Work out the finished part from the listing and answer in its coordinate system (mm). A direction names the side the tool comes from. Give positions to 0.01 mm unless a question says otherwise; leave off trailing zeros. Write each loop counter-clockwise with the first axis right and the second up, starting at its lowest first coordinate (ties: lowest second). Pieces come first, ordered by that corner, then holes. Notation, with made-up numbers: (34, 28) -> (87, 28) arc R25 cw to (87, 65) -> close; hole circle Ø8 at (34.5, -22.75). An arc over 180 degrees is marked (long way). Use a Markdown table: item, result. Add a question column.
Q1. Section D-D, the plane z = 5 is taken. Give the vertices of the cut face in (x, y).
Q2. Consider line 1 (X direction, y = 2.3, z = 5); line 2 (X direction, y = 2.35, z = 35); line 3 (X direction, y = 1, z = 43.5). Determine where each line is inside the solid, lowest interval first.
Q3. Section B-B, the plane z = 27.5 is taken. Give the vertices of the cut face in (x, y), plus the area to 4 significant figures.
Q4. Each of these flat-tipped pins is pushed along its axis until it touches: pin 1 Ø2.5 at (x, z) = (-40, 5) entering from +Y; pin 2 Ø1 at (x, y) = (9, 0.5) entering from +Z; pin 3 Ø2 at (y, z) = (1.5, 47.5) entering from +X. Where does it stop, or does it pass through?
Q5. For faces 5 (the face through (-40, 2, 47)), 6 (the face through (42, 2, 49.25)), 7 (the face through (0, 2, 20)), determine the directions among +Z, -Z, +X, -X, +Y, -Y from which every point of the face is accessible in a straight line to the end or side of a thin tool.
Q6. Section C-C, the plane y = 2.5 is taken. State how many separate pieces and enclosed holes the cut face has, plus the area to 3 significant figures.
Q7. For a pull along Z with two mould halves and no side action, classify faces 1 (the face through (31.4, 2.28, 4.94)), 2 (the face through (45, 2, 52)), 3 (the face through (-30.18, 2.28, 33.61)), 4 (the face through (26.5, 2.3, 21)) as pulls with the +Z half, pulls with the -Z half, needs draft (parallel to the pull), parting line crosses it, or undercut.
Q8. Section A-A, the plane x = -30 is taken. Give the vertices of the cut face in (y, z), plus the area to 3 significant figures.
from build123d import *

# Parameters (mm, degrees)
SKETCH1_W           = 90
SKETCH1_H           = 55
SKETCH1_R           = 1.45
BOSS_EXTRUDE1_DEPTH = 4.5
SKETCH2_W           = 55
SKETCH2_H           = 35
CUT_EXTRUDE1_DEPTH  = 5.5
SKETCH3_W           = 5
SKETCH3_H           = 4.25
CUT_EXTRUDE2_DEPTH  = 5.5
SKETCH4_R           = 1.4
CUT_EXTRUDE3_DEPTH  = 5.5
CHAMFER1_SIZE       = 5
CHAMFER2_SIZE       = 2


with BuildPart() as part:
    # Sketch1 → Boss-Extrude1 (new body)
    with BuildSketch(Plane(origin=(0, 0, 0), x_dir=(1, 0, 0), z_dir=(0, 1, 0))):
        with Locations((0, -27.5)):
            Rectangle(SKETCH1_W, SKETCH1_H)
        with Locations((-40, -40)):
            Circle(SKETCH1_R, mode=Mode.SUBTRACT)
        with Locations((-40, -5)):
            Circle(SKETCH1_R, mode=Mode.SUBTRACT)
        with Locations((40, -40)):
            Circle(SKETCH1_R, mode=Mode.SUBTRACT)
        with Locations((40, -5)):
            Circle(SKETCH1_R, mode=Mode.SUBTRACT)
    extrude(amount=BOSS_EXTRUDE1_DEPTH)

    # Sketch2 → Cut-Extrude1 (cut, through all)
    with BuildSketch(Plane(origin=(0, 4.5, 0), x_dir=(1, 0, 0), z_dir=(0, 1, 0))):
        with Locations((0, -37.5)):
            Rectangle(SKETCH2_W, SKETCH2_H)
    extrude(amount=-CUT_EXTRUDE1_DEPTH, mode=Mode.SUBTRACT)

    # Sketch3 → Cut-Extrude2 (cut, through all)
    with BuildSketch(Plane(origin=(0, 4.5, 0), x_dir=(1, 0, 0), z_dir=(0, 1, 0))):
        with Locations((-42.5, -47.125)):
            Rectangle(SKETCH3_W, SKETCH3_H)
        with Locations((42.5, -47.125)):
            Rectangle(SKETCH3_W, SKETCH3_H)
    extrude(amount=-CUT_EXTRUDE2_DEPTH, mode=Mode.SUBTRACT)

    # Sketch4 → Cut-Extrude3 (cut, through all)
    with BuildSketch(Plane(origin=(0, 4.5, 0), x_dir=(1, 0, 0), z_dir=(0, 1, 0))):
        with Locations((-30, -35)):
            Circle(SKETCH4_R)
        with Locations((-30, -5)):
            Circle(SKETCH4_R)
    cut_extrude3 = extrude(amount=-CUT_EXTRUDE3_DEPTH, mode=Mode.SUBTRACT)

    # Mirror1: Cut-Extrude3 across plane
    add(cut_extrude3.mirror(Plane(origin=(0, 0, 0), x_dir=(0, 0, 1), z_dir=(1, 0, 0))), mode=Mode.SUBTRACT)

    # Chamfer1
    chamfer1_edges = [part.edges().sort_by_distance(p)[0] for p in [
        (27.5, 2.25, 55),
        (-27.5, 2.25, 55),
    ]]
    chamfer(chamfer1_edges, length=CHAMFER1_SIZE)

    # Chamfer2
    chamfer2_edges = [part.edges().sort_by_distance(p)[0] for p in [
        (27.5, 2.25, 20),
        (-27.5, 2.25, 20),
    ]]
    chamfer(chamfer2_edges, length=CHAMFER2_SIZE)


solid = part.part
Result set:
| question | item | result |
|---|---|---|
| 1 | outline | (-45, 0) -> (-41.45, 0) -> (-41.45, 4.5) -> (-45, 4.5) -> close; (-38.55, 0) -> (-31.4, 0) -> (-31.4, 4.5) -> (-38.55, 4.5) -> close; (-28.6, 0) -> (28.6, 0) -> (28.6, 4.5) -> (-28.6, 4.5) -> close; (31.4, 0) -> (38.55, 0) -> (38.55, 4.5) -> (31.4, 4.5) -> close; (41.45, 0) -> (45, 0) -> (45, 4.5) -> (41.45, 4.5) -> close |
| 2 | line 1 | x = -45 to -41.45, -38.55 to -31.4, -28.6 to 28.6, 31.4 to 38.55, 41.45 to 45 |
| 2 | line 2 | x = -45 to -31.4, -28.6 to -27.5, 27.5 to 28.6, 31.4 to 45 |
| 2 | line 3 | x = -45 to -27.5, 27.5 to 45 |
| 3 | outline | (-45, 0) -> (-27.5, 0) -> (-27.5, 4.5) -> (-45, 4.5) -> close; (27.5, 0) -> (45, 0) -> (45, 4.5) -> (27.5, 4.5) -> close |
| 3 | area | 157.5 mm2 |
| 4 | pin 1 | passes through |
| 4 | pin 2 | stops at z = 20 |
| 4 | pin 3 | stops at x = 40 |
| 5 | face 5 | -X, +Y, -Y |
| 5 | face 6 | +X, +Y, -Y |
| 5 | face 7 | +Z, +Y, -Y |
| 6 | separate pieces | 1 |
| 6 | enclosed holes | 8 |
| 6 | area | 2,910 mm2 |
| 7 | face 1 | undercut |
| 7 | face 2 | needs draft |
| 7 | face 3 | undercut |
| 7 | face 4 | pulls with the +Z half |
| 8 | outline | (0, 0) -> (4.5, 0) -> (4.5, 3.6) -> (0, 3.6) -> close; (0, 6.4) -> (4.5, 6.4) -> (4.5, 33.6) -> (0, 33.6) -> close; (0, 36.4) -> (4.5, 36.4) -> (4.5, 52.5) -> (0, 52.5) -> close |
| 8 | area | 211 mm2 |
